Here's how the part is built. I have some questions about the finished solid (model axes, mm). A direction names the side the tool comes from. Round coordinates to 2 decimals unless told otherwise and drop trailing zeros. Order: outer loops, then holes, each group sorted by start corner. A loop starts at its lowest first (then second) coordinate and runs counter-clockwise, first axis right, second up. Notation, with made-up numbers: (34, -16.5) -> (66, -16.5) arc R27 ccw to (66, 10.5) -> close; hole circle Ø9 at (28, 22). An arc over 180 degrees is marked (long way). Use a Markdown table: item, result. Add a question column.
from build123d import *

# Parameters (mm, degrees)
SKETCH1_W            = 50
SKETCH1_H            = 75
BOSS_EXTRUDE1_DEPTH  = 2
SKETCH2_W            = 50
SKETCH2_H            = 40
BOSS_EXTRUDE2_DEPTH  = 15
CUT_EXTRUDE1_DEPTH   = 40
SKETCH4_W            = 30
SKETCH4_H            = 10
BOSS_EXTRUDE3_DEPTH  = 15
CUT_EXTRUDE2_DEPTH   = 30
SKETCH6_R            = 4.75
BOSS_EXTRUDE6_DEPTH  = 17
SKETCH7_W            = 9.72
SKETCH7_H            = 16
BOSS_EXTRUDE9_DEPTH  = 5.5
SKETCH8_W            = 9
SKETCH8_H            = 3
BOSS_EXTRUDE10_DEPTH = 5
SKETCH9_R            = 1.75
CUT_EXTRUDE4_DEPTH   = 2


with BuildPart() as part:
    # Sketch1 → Boss-Extrude1 (new body)
    with BuildSketch(Plane(origin=(0, 0, 0), x_dir=(1, 0, 0), z_dir=(0, 1, 0))):
        Rectangle(SKETCH1_W, SKETCH1_H)
    extrude(amount=BOSS_EXTRUDE1_DEPTH)

    # Sketch2 → Boss-Extrude2 (add)
    with BuildSketch(Plane(origin=(0, 2, 0), x_dir=(1, 0, 0), z_dir=(0, 1, 0))):
        with Locations((0, 12)):
            Rectangle(SKETCH2_W, SKETCH2_H)
    extrude(amount=BOSS_EXTRUDE2_DEPTH)

    # Sketch3 → Cut-Extrude1 (cut)
    with BuildSketch(Plane(origin=(0, 0, -32), x_dir=(-1, 0, 0), z_dir=(0, 0, -1))):
        with BuildLine():
            Line((4.025, 25), (4.025, 6.1))
            ThreePointArc((4.025, 6.1), (3.702817459, 5.322182541), (2.925, 5))
            Line((2.925, 5), (2.875, 5))
            ThreePointArc((2.875, 5), (2.097182541, 5.322182541), (1.775, 6.1))
            Line((1.775, 6.1), (1.775, 25))
            Line((1.775, 25), (4.025, 25))
        make_face()
        with BuildLine():
            Line((-1.125, 25), (1.125, 25))
            Line((1.125, 25), (1.125, 6.1))
            ThreePointArc((1.125, 6.1), (0.802817459, 5.322182541), (0.025, 5))
            Line((0.025, 5), (-0.025, 5))
            ThreePointArc((-0.025, 5), (-0.802817459, 5.322182541), (-1.125, 6.1))
            Line((-1.125, 6.1), (-1.125, 25))
        make_face()
        with BuildLine():
            Line((6.925, 25), (6.925, 6.1))
            ThreePointArc((6.925, 6.1), (6.602817459, 5.322182541), (5.825, 5))
            Line((5.825, 5), (5.775, 5))
            ThreePointArc((5.775, 5), (4.997182541, 5.322182541), (4.675, 6.1))
            Line((4.675, 6.1), (4.675, 25))
            Line((4.675, 25), (6.925, 25))
        make_face()
        with BuildLine():
            Line((9.825, 25), (9.825, 6.1))
            ThreePointArc((9.825, 6.1), (9.502817459, 5.322182541), (8.725, 5))
            Line((8.725, 5), (8.675, 5))
            ThreePointArc((8.675, 5), (7.897182541, 5.322182541), (7.575, 6.1))
            Line((7.575, 6.1), (7.575, 25))
            Line((7.575, 25), (9.825, 25))
        make_face()
        with BuildLine():
            Line((12.725, 25), (12.725, 6.1))
            ThreePointArc((12.725, 6.1), (12.402817459, 5.322182541), (11.625, 5))
            Line((11.625, 5), (11.575, 5))
            ThreePointArc((11.575, 5), (10.797182541, 5.322182541), (10.475, 6.1))
            Line((10.475, 6.1), (10.475, 25))
            Line((10.475, 25), (12.725, 25))
        make_face()
        with BuildLine():
            Line((15.625, 25), (15.625, 6.1))
            ThreePointArc((15.625, 6.1), (15.302817459, 5.322182541), (14.525, 5))
            Line((14.525, 5), (14.475, 5))
            ThreePointArc((14.475, 5), (13.697182541, 5.322182541), (13.375, 6.1))
            Line((13.375, 6.1), (13.375, 25))
            Line((13.375, 25), (15.625, 25))
        make_face()
        with BuildLine():
            Line((18.525, 25), (18.525, 6.1))
            ThreePointArc((18.525, 6.1), (18.202817459, 5.322182541), (17.425, 5))
            Line((17.425, 5), (17.375, 5))
            ThreePointArc((17.375, 5), (16.597182541, 5.322182541), (16.275, 6.1))
            Line((16.275, 6.1), (16.275, 25))
            Line((16.275, 25), (18.525, 25))
        make_face()
        with BuildLine():
            Line((21.425, 25), (21.425, 6.1))
            ThreePointArc((21.425, 6.1), (21.102817459, 5.322182541), (20.325, 5))
            Line((20.325, 5), (20.275, 5))
            ThreePointArc((20.275, 5), (19.497182541, 5.322182541), (19.175, 6.1))
            Line((19.175, 6.1), (19.175, 25))
            Line((19.175, 25), (21.425, 25))
        make_face()
        with BuildLine():
            Line((24.325, 25), (24.325, 6.1))
            ThreePointArc((24.325, 6.1), (24.002817459, 5.322182541), (23.225, 5))
            Line((23.225, 5), (23.175, 5))
            ThreePointArc((23.175, 5), (22.397182541, 5.322182541), (22.075, 6.1))
            Line((22.075, 6.1), (22.075, 25))
            Line((22.075, 25), (24.325, 25))
        make_face()
        with BuildLine():
            Line((-1.775, 25), (-1.775, 6.1))
            ThreePointArc((-1.775, 6.1), (-2.097182541, 5.322182541), (-2.875, 5))
            Line((-2.875, 5), (-2.925, 5))
            ThreePointArc((-2.925, 5), (-3.702817459, 5.322182541), (-4.025, 6.1))
            Line((-4.025, 6.1), (-4.025, 25))
            Line((-4.025, 25), (-1.775, 25))
        make_face()
        with BuildLine():
            Line((-4.675, 25), (-4.675, 6.1))
            ThreePointArc((-4.675, 6.1), (-4.997182541, 5.322182541), (-5.775, 5))
            Line((-5.775, 5), (-5.825, 5))
            ThreePointArc((-5.825, 5), (-6.602817459, 5.322182541), (-6.925, 6.1))
            Line((-6.925, 6.1), (-6.925, 25))
            Line((-6.925, 25), (-4.675, 25))
        make_face()
        with BuildLine():
            Line((-7.575, 25), (-7.575, 6.1))
            ThreePointArc((-7.575, 6.1), (-7.897182541, 5.322182541), (-8.675, 5))
            Line((-8.675, 5), (-8.725, 5))
            ThreePointArc((-8.725, 5), (-9.502817459, 5.322182541), (-9.825, 6.1))
            Line((-9.825, 6.1), (-9.825, 25))
            Line((-9.825, 25), (-7.575, 25))
        make_face()
        with BuildLine():
            Line((-10.475, 25), (-10.475, 6.1))
            ThreePointArc((-10.475, 6.1), (-10.797182541, 5.322182541), (-11.575, 5))
            Line((-11.575, 5), (-11.625, 5))
            ThreePointArc((-11.625, 5), (-12.402817459, 5.322182541), (-12.725, 6.1))
            Line((-12.725, 6.1), (-12.725, 25))
            Line((-12.725, 25), (-10.475, 25))
        make_face()
        with BuildLine():
            Line((-13.375, 25), (-13.375, 6.1))
            ThreePointArc((-13.375, 6.1), (-13.697182541, 5.322182541), (-14.475, 5))
            Line((-14.475, 5), (-14.525, 5))
            ThreePointArc((-14.525, 5), (-15.302817459, 5.322182541), (-15.625, 6.1))
            Line((-15.625, 6.1), (-15.625, 25))
            Line((-15.625, 25), (-13.375, 25))
        make_face()
        with BuildLine():
            Line((-16.275, 25), (-16.275, 6.1))
            ThreePointArc((-16.275, 6.1), (-16.597182541, 5.322182541), (-17.375, 5))
            Line((-17.375, 5), (-17.425, 5))
            ThreePointArc((-17.425, 5), (-18.202817459, 5.322182541), (-18.525, 6.1))
            Line((-18.525, 6.1), (-18.525, 25))
            Line((-18.525, 25), (-16.275, 25))
        make_face()
        with BuildLine():
            Line((-19.175, 25), (-19.175, 6.1))
            ThreePointArc((-19.175, 6.1), (-19.497182541, 5.322182541), (-20.275, 5))
            Line((-20.275, 5), (-20.325, 5))
            ThreePointArc((-20.325, 5), (-21.102817459, 5.322182541), (-21.425, 6.1))
            Line((-21.425, 6.1), (-21.425, 25))
            Line((-21.425, 25), (-19.175, 25))
        make_face()
        with BuildLine():
            Line((-22.075, 25), (-22.075, 6.1))
            ThreePointArc((-22.075, 6.1), (-22.397182541, 5.322182541), (-23.175, 5))
            Line((-23.175, 5), (-23.225, 5))
            ThreePointArc((-23.225, 5), (-24.002817459, 5.322182541), (-24.325, 6.1))
            Line((-24.325, 6.1), (-24.325, 25))
            Line((-24.325, 25), (-22.075, 25))
        make_face()
    extrude(amount=-CUT_EXTRUDE1_DEPTH, mode=Mode.SUBTRACT)

    # Sketch4 → Boss-Extrude3 (add)
    with BuildSketch(Plane.XZ):
        with Locations((0, 32.5)):
            Rectangle(SKETCH4_W, SKETCH4_H)
        with Locations((0, -32.5)):
            Rectangle(SKETCH4_W, SKETCH4_H)
    extrude(amount=BOSS_EXTRUDE3_DEPTH)

    # Sketch5 → Cut-Extrude2 (cut)
    with BuildSketch(Plane.ZY.offset(15)):
        Polygon((-27.5, -15), (-27.5, -5), (-32.5, -15), align=None)
        Polygon((32.5, -15), (27.5, -15), (27.5, -5), align=None)
    extrude(amount=-CUT_EXTRUDE2_DEPTH, mode=Mode.SUBTRACT)

    # Sketch6 → Boss-Extrude6 (add)
    with BuildSketch(Plane.XZ):
        with Locations(Location((-20, -27.5, 0), (0, 0, 90))):
            Circle(SKETCH6_R)
    extrude(amount=BOSS_EXTRUDE6_DEPTH)

    # Sketch7 → Boss-Extrude9 (add)
    with BuildSketch(Plane.XZ):
        with Locations((20.14, 19.274770973)):
            Rectangle(SKETCH7_W, SKETCH7_H)
    extrude(amount=BOSS_EXTRUDE9_DEPTH)

    # Sketch8 → Boss-Extrude10 (add)
    with BuildSketch(Plane(origin=(0, 0, 0), x_dir=(-1, 0, 0), z_dir=(0, -1, 0))):
        with Locations((-20.14, -3.274770973)):
            Rectangle(SKETCH8_W, SKETCH8_H)
        with Locations((-20.14, -8.274770973)):
            Rectangle(SKETCH8_W, SKETCH8_H)
        with Locations((-20.14, 1.725229027)):
            Rectangle(SKETCH8_W, SKETCH8_H)
    extrude(amount=BOSS_EXTRUDE10_DEPTH)

    # Sketch9 → Cut-Extrude4 (cut)
    with BuildSketch(Plane(origin=(0, 2, 0), x_dir=(1, 0, 0), z_dir=(0, 1, 0))):
        with Locations(Location((-21.25, 34.5, 0), (0, 0, 270))):
            Circle(SKETCH9_R)
        with Locations(Location((21.25, 34.5, 0), (0, 0, 270))):
            Circle(SKETCH9_R)
        with Locations(Location((-21.25, -34.5, 0), (0, 0, 270))):
            Circle(SKETCH9_R)
        with Locations(Location((21.25, -34.5, 0), (0, 0, 270))):
            Circle(SKETCH9_R)
    extrude(amount=-CUT_EXTRUDE4_DEPTH, mode=Mode.SUBTRACT)


solid = part.part
(1) I'm going to push flat-ended pins straight in: P1, Ø8, axis at x = -4, z = -29, coming from the -Y side; P2, Ø4.5, axis at x = -21.25, z = 34.5, coming from the +Y side. Where does each tip first touch, or does it pass through?
(2) On a 3-axis mill with a long thin cutter (end or side, diameter ignored), from which of +Z, -Z, +X, -X, +Y, -Y can I reach the whole of each face in a straight line? I mean faces 1 (the flat face through (24.325, 11, -12)), 2 (the flat face through (0, -2, -27.5)), 3 (the flat face through (15.28, -3, 19)). Say none if no direction works.
(3) Please list where these lines run through material, in increasing order: probe 1 along Z at (x, y) = (22, -0.5); probe 2 along X at (y, z) = (1.45, -34.5); probe 3 along X at (y, z) = (1, -34). Write a range as from..to.
(4) I want a section at A-A on y = -14. List the corners of the cut face in (x, z) for me, and give its area (3 significant figures).
(5) I want a section at C-C on y = 7. State how many separate pieces and enclosed holes the cut face has, and give its area (3 significant figures).
(6) I want a section at B-B on z = 34.5. List the corners of the cut face in (x, y) for me.
(7) If we mould it in two halves opening along X, with no side actions, what happens to faces 4 (the flat face through (15, -7, 34)), 5 (the flat face through (-22.075, 11, -12)), 6 (the flat face through (-18.525, 12, -12)), 7 (the flat face through (-2, 4, -32))? For each: pulls with the +X half, pulls with the -X half, needs draft (parallel to the pull), parting line crosses it, or undercut.
Output:
| question | item | result |
|---|---|---|
| 1 | P1 | y = -15 |
| 1 | P2 | y = 2 |
| 2 | face 1 | +Z, -Z, +Y |
| 2 | face 2 | +X, -Y |
| 2 | face 3 | +Z, -Z, -X, -Y |
| 3 | probe 1 | -3.23..-0.23, 1.77..4.77, 6.77..9.77, 11.27..27.27 |
| 3 | probe 2 | -25..-23, -19.5..19.5, 23..25 |
| 3 | probe 3 | -25..-22.93, -19.57..19.57, 22.93..25 |
| 4 | outline | circle Ø9.5 at (-20, -27.5); (-15, -37.5) -> (15, -37.5) -> (15, -32) -> (-15, -32) -> close; (-15, 32) -> (15, 32) -> (15, 37.5) -> (-15, 37.5) -> close |
| 4 | area | 401 mm² |
| 5 | separate pieces | 18 |
| 5 | enclosed holes | 0 |
| 5 | area | 470 mm² |
| 6 | outline | (-25, 0) -> (-23, 0) -> (-23, 2) -> (-25, 2) -> close; (-19.5, 0) -> (-15, 0) -> (-15, -15) -> (15, -15) -> (15, 0) -> (19.5, 0) -> (19.5, 2) -> (-19.5, 2) -> close; (23, 0) -> (25, 0) -> (25, 2) -> (23, 2) -> close |
| 7 | face 4 | pulls with the +X half |
| 7 | face 5 | undercut |
| 7 | face 6 | undercut |
| 7 | face 7 | needs draft |
